Build history of the part. All positions in model axes, mm. Face numbers are marked on the shaded views. A direction names the side the tool comes from. Coordinates: 2 decimals unless noted, no trailing zeros. Order: outer loops, then holes, each group sorted by start corner. A loop starts at its lowest first (then second) coordinate and runs counter-clockwise, first axis right, second up. Notation, with made-up numbers: M 51,-27 L 99,-27 A19 ccw 99,3 Z; hole C 37,64 d2. An arc over 180 degrees is marked long. Write item = value, one per line. Start each with the question number.
Q1. Band-saw the part on D-D on z = 9.5. Write the cut outline in (x, y).
Q2. Band-saw the part on A-A on z = 44. Write the cut outline in (x, y) (3 decimals), plus the area to 3 significant figures.
Q3. Pull direction Y, two halves, no side cores. Call the marked faces 1, 2 and 3: released by +Y, released by -Y, zero draft, split by the parting line, or undercut.
Q4. Band-saw the part on B-B on y = -44. Write the cut outline in (x, z), plus the area to 3 significant figures.
Q5. Drill centre lines: probe 1 along Z at (x, y) = (11, -39); probe 2 along Y at (x, z) = (11.5, 41) (3 decimals); probe 3 along Y at (x, z) = (17.5, 12.5). Where is each one in solid material? Low to high.
Q6. 3-axis set-ups, long thin cutter, end or side, ignore diameter. For the marked faces 4, 5 and 6: which of +Z, -Z, +X, -X, +Y, -Y reach the whole face in a straight line?
Q7. Band-saw the part on C-C on x = -61. Write the cut outline in (y, z), plus the area to 3 significant figures.
Q8. Pin check, flat tips, straight feed: P1, Ø6, axis at x = -7, z = 45, coming from the -Y side (3 decimals); P2, Ø5, axis at y = -137.5, z = 39.5, coming from the -X side. Stop position of each tip, or through.
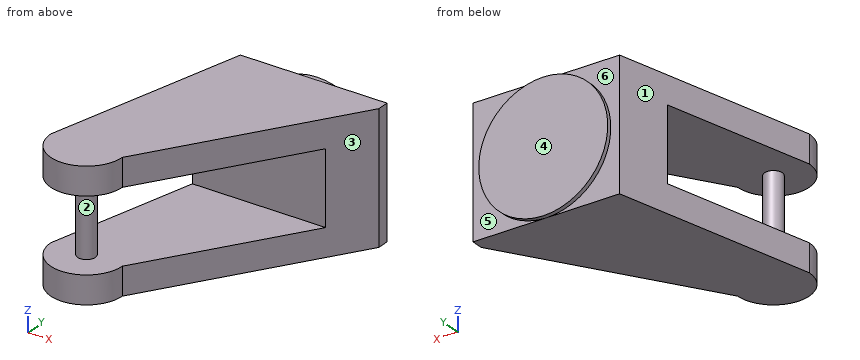
```python
from build123d import *

# Parameters (mm, degrees)
ESTRUSIONE_ESTRUSIONE1_DEPTH  = 88
TAGLIO_ESTRUSIONE2_DEPTH      = 200.184672352
TAGLIO_ESTRUSIONE2_DEPTH_BACK = 200.184672352
SCHIZZO4_R                    = 6.05
ESTRUSIONE_ESTRUSIONE2_DEPTH  = 69
SCHIZZO6_R                    = 44
ESTRUSIONE_ESTRUSIONE3_DEPTH  = 3


with BuildPart() as part:
    # Schizzo1 → Estrusione-Estrusione1 (new body)
    with BuildSketch(Plane.XY):
        with BuildLine():
            Line((-50, 4), (-83.39, -133.65))
            ThreePointArc((-83.39, -133.65), (-59, -158.04), (-34.61, -133.65))
            Line((-34.61, -133.65), (50, -4))
            Line((50, -4), (50, 4))
            Line((50, 4), (-50, 4))
        make_face()
    extrude(amount=ESTRUSIONE_ESTRUSIONE1_DEPTH)

    # Schizzo2 → Taglio-Estrusione2 (cut, two sides: drawn at the far end of the back side and taken through both)
    with BuildSketch(Plane(origin=(0, 0, 0), x_dir=(0, 0, -1), z_dir=(1, 0, 0)).offset(-TAGLIO_ESTRUSIONE2_DEPTH_BACK)):
        Polygon((-69, -45.845), (-69, -245.845), (-19, -245.845), (-19, -45.845), (-19, -30.845), (-69, -30.845), align=None)
    extrude(amount=TAGLIO_ESTRUSIONE2_DEPTH + TAGLIO_ESTRUSIONE2_DEPTH_BACK, mode=Mode.SUBTRACT)

    # Schizzo4 → Estrusione-Estrusione2 (add)
    with BuildSketch(Plane.XY.offset(88)):
        with Locations(Location((-59, -133.65, 0), (0, 0, 270))):
            Circle(SCHIZZO4_R)
    extrude(amount=-ESTRUSIONE_ESTRUSIONE2_DEPTH)

    # Schizzo6 → Estrusione-Estrusione3 (add)
    with BuildSketch(Plane(origin=(0, 4, 0), x_dir=(1, 0, 0), z_dir=(0, 1, 0))):
        with Locations(Location((0, -44, 0), (0, 0, 90))):
            Circle(SCHIZZO6_R)
    extrude(amount=ESTRUSIONE_ESTRUSIONE3_DEPTH)


solid = part.part
```
Recorded:
q1.outline = M -83.39,-133.65 A24.39 ccw -34.61,-133.65 L 50,-4 L 50,4 L 27.31,4 L 27.31,7 L -27.31,7 L -27.31,4 L -50,4 Z
q2.outline = C -59,-133.65 d12.1; M -58.452,-30.845 L 32.481,-30.845 L 50,-4 L 50,4 L 44,4 L 44,7 L -44,7 L -44,4 L -50,4 Z
q2.area = 3,780 mm2
q3.face_1 = released by +Y
q3.face_2 = undercut
q3.face_3 = released by -Y
q4.outline = M -61.64,0 L 23.9,0 L 23.9,19 L -61.64,19 Z; M -61.64,69 L 23.9,69 L 23.9,88 L -61.64,88 Z
q4.area = 3,250 mm2
q5.probe_1 = 0 to 19, 69 to 88
q5.probe_2 = -30.845 to 7
q5.probe_3 = -53.8 to 7
q6.face_4 = +Z, -Z, +X, -X, +Y
q6.face_5 = +X, +Y
q6.face_6 = -X, +Y
q7.outline = M -157.96,0 L -41.35,0 L -41.35,19 L -127.94,19 L -127.94,69 L -41.35,69 L -41.35,88 L -157.96,88 L -157.96,69 L -139.36,69 L -139.36,19 L -157.96,19 Z
q7.area = 5,000 mm2
q8.P1 = -30.845
q8.P2 = -64.9
